from build123d import *

# Parameters (mm, degrees)
ESBO_O1_W                = 3
ESBO_O1_H                = 3
RESSALTO_EXTRUS_O1_DEPTH = 230


with BuildPart() as part:
    # Esboço1 → Ressalto-extrusão1 (new, symmetric)
    with BuildSketch(Plane.XY):
        with BuildLine():
            Line((15, 13.5), (15, 4.05))
            Line((15, 4.05), (13, 4.05))
            Line((13, 4.05), (13, 9))
            Line((13, 9), (10.414213562, 9))
            Line((10.414213562, 9), (7.9, 6.485786438))
            Line((7.9, 6.485786438), (7.9, -7.36e-07))
            Line((7.9, -7.36e-07), (7.9, -6.485786438))
            Line((7.9, -6.485786438), (10.414213562, -9))
            Line((10.414213562, -9), (13, -9))
            Line((13, -9), (13, -4.05))
            Line((13, -4.05), (15, -4.05))
            Line((15, -4.05), (15, -13.5))
            ThreePointArc((15, -13.5), (14.560660172, -14.560660172), (13.5, -15))
            Line((13.5, -15), (4.05, -15))
            Line((4.05, -15), (4.05, -13))
            Line((4.05, -13), (9, -13))
            Line((9, -13), (9, -10.414213562))
            Line((9, -10.414213562), (6.485786438, -7.9))
            Line((6.485786438, -7.9), (-7.36e-07, -7.9))
            Line((-7.36e-07, -7.9), (-6.485786438, -7.9))
            Line((-6.485786438, -7.9), (-9, -10.414213562))
            Line((-9, -10.414213562), (-9, -13))
            Line((-9, -13), (-4.05, -13))
            Line((-4.05, -13), (-4.05, -15))
            Line((-4.05, -15), (-13.5, -15))
            ThreePointArc((-13.5, -15), (-14.560660172, -14.560660172), (-15, -13.5))
            Line((-15, -13.5), (-15, -4.05))
            Line((-15, -4.05), (-13, -4.05))
            Line((-13, -4.05), (-13, -9))
            Line((-13, -9), (-10.414213562, -9))
            Line((-10.414213562, -9), (-7.9, -6.485786438))
            Line((-7.9, -6.485786438), (-7.9, 7.36e-07))
            Line((-7.9, 7.36e-07), (-7.9, 6.485786438))
            Line((-7.9, 6.485786438), (-10.414213562, 9))
            Line((-10.414213562, 9), (-13, 9))
            Line((-13, 9), (-13, 4.05))
            Line((-13, 4.05), (-15, 4.05))
            Line((-15, 4.05), (-15, 13.5))
            ThreePointArc((-15, 13.5), (-14.560660172, 14.560660172), (-13.5, 15))
            Line((-13.5, 15), (-4.05, 15))
            Line((-4.05, 15), (-4.05, 13))
            Line((-4.05, 13), (-9, 13))
            Line((-9, 13), (-9, 10.414213562))
            Line((-9, 10.414213562), (-6.485786438, 7.9))
            Line((-6.485786438, 7.9), (7.36e-07, 7.9))
            Line((7.36e-07, 7.9), (6.485786438, 7.9))
            Line((6.485786438, 7.9), (9, 10.414213562))
            Line((9, 10.414213562), (9, 13))
            Line((9, 13), (4.05, 13))
            Line((4.05, 13), (4.05, 15))
            Line((4.05, 15), (13.5, 15))
            ThreePointArc((13.5, 15), (14.560660172, 14.560660172), (15, 13.5))
        make_face()
        with Locations((-11.5, 11.5)):
            Rectangle(ESBO_O1_W, ESBO_O1_H, mode=Mode.SUBTRACT)
        with BuildLine():
            Line((-6.9, 1.000000736), (-6.9, 7.36e-07))
            Line((-6.9, 7.36e-07), (-6.9, -1.000000736))
            Line((-6.9, -1.000000736), (-5.966782929, -1.000000736))
            ThreePointArc((-5.966782929, -1.000000736), (-5.665339038, -2.122836212), (-5.154690025, -3.167281286))
            Line((-5.154690025, -3.167281286), (-6.9, -4.91259126))
            Line((-6.9, -4.91259126), (-6.9, -5.827922061))
            Line((-6.9, -5.827922061), (-5.827922061, -6.9))
            Line((-5.827922061, -6.9), (-4.91259126, -6.9))
            Line((-4.91259126, -6.9), (-3.167281286, -5.154690025))
            ThreePointArc((-3.167281286, -5.154690025), (-2.122836212, -5.665339038), (-1.000000736, -5.966782929))
            Line((-1.000000736, -5.966782929), (-1.000000736, -6.9))
            Line((-1.000000736, -6.9), (-7.36e-07, -6.9))
            Line((-7.36e-07, -6.9), (1.000000736, -6.9))
            Line((1.000000736, -6.9), (1.000000736, -5.966782929))
            ThreePointArc((1.000000736, -5.966782929), (2.122836212, -5.665339038), (3.167281286, -5.154690025))
            Line((3.167281286, -5.154690025), (4.91259126, -6.9))
            Line((4.91259126, -6.9), (5.827922061, -6.9))
            Line((5.827922061, -6.9), (6.9, -5.827922061))
            Line((6.9, -5.827922061), (6.9, -4.91259126))
            Line((6.9, -4.91259126), (5.154690025, -3.167281286))
            ThreePointArc((5.154690025, -3.167281286), (5.665339038, -2.122836212), (5.966782929, -1.000000736))
            Line((5.966782929, -1.000000736), (6.9, -1.000000736))
            Line((6.9, -1.000000736), (6.9, -7.36e-07))
            Line((6.9, -7.36e-07), (6.9, 1.000000736))
            Line((6.9, 1.000000736), (5.966782929, 1.000000736))
            ThreePointArc((5.966782929, 1.000000736), (5.665339038, 2.122836212), (5.154690025, 3.167281286))
            Line((5.154690025, 3.167281286), (6.9, 4.91259126))
            Line((6.9, 4.91259126), (6.9, 5.827922061))
            Line((6.9, 5.827922061), (5.827922061, 6.9))
            Line((5.827922061, 6.9), (4.91259126, 6.9))
            Line((4.91259126, 6.9), (3.167281286, 5.154690025))
            ThreePointArc((3.167281286, 5.154690025), (2.122836212, 5.665339038), (1.000000736, 5.966782929))
            Line((1.000000736, 5.966782929), (1.000000736, 6.9))
            Line((1.000000736, 6.9), (7.36e-07, 6.9))
            Line((7.36e-07, 6.9), (-1.000000736, 6.9))
            Line((-1.000000736, 6.9), (-1.000000736, 5.966782929))
            ThreePointArc((-1.000000736, 5.966782929), (-2.122836212, 5.665339038), (-3.167281286, 5.154690025))
            Line((-3.167281286, 5.154690025), (-4.91259126, 6.9))
            Line((-4.91259126, 6.9), (-5.827922061, 6.9))
            Line((-5.827922061, 6.9), (-6.9, 5.827922061))
            Line((-6.9, 5.827922061), (-6.9, 4.91259126))
            Line((-6.9, 4.91259126), (-5.154690025, 3.167281286))
            ThreePointArc((-5.154690025, 3.167281286), (-5.665339038, 2.122836212), (-5.966782929, 1.000000736))
            Line((-5.966782929, 1.000000736), (-6.9, 1.000000736))
        make_face(mode=Mode.SUBTRACT)
        with Locations((11.5, 11.5)):
            Rectangle(ESBO_O1_W, ESBO_O1_H, mode=Mode.SUBTRACT)
        with Locations((11.5, -11.5)):
            Rectangle(ESBO_O1_W, ESBO_O1_H, mode=Mode.SUBTRACT)
        with Locations((-11.5, -11.5)):
            Rectangle(ESBO_O1_W, ESBO_O1_H, mode=Mode.SUBTRACT)
    extrude(amount=RESSALTO_EXTRUS_O1_DEPTH, both=True)


solid = part.part
Geometry check sheet. Reference: the model listing, model coordinates, mm. A direction names the side the tool comes from. Round coordinates to 2 decimals unless told otherwise and drop trailing zeros. Use one line per item in the form item = value.
1. Scan lines: line 1 along Y through (x, z) = (12.75, -48); line 2 along X through (y, z) = (-7.5, -74). Record each from-to range of solid material in increasing order. Write a range as from..to.
Working result:
line_1 = -15..-13, -10..-9, 9..10, 13..15
line_2 = -15..-13, -8.91..8.91, 13..15
2. Cross-section at A-A, the plane z = 196. Count the separate pieces of the cut face and the enclosed holes in it, plus the area to 3 significant figures.
Working result:
separate_pieces = 1
enclosed_holes = 5
area = 301 mm^2
3. Go/stop test with flat-tipped pins: pin 1 (1.6 mm diameter, centred on x = 14, z = 30.5, fed in from +Y); pin 2 (1.5 mm diameter, centred on y = 1.5, z = 178, fed in from -X); pin 3 (2 mm diameter, centred on x = -1.5, z = -51.5, fed in from +Y); pin 4 (4 mm diameter, centred on y = -0.5, z = -96.5, fed in from +X). Record where each tip stops, or that it passes through.
Working result:
pin_1 = 15
pin_2 = -7.9
pin_3 = 7.9
pin_4 = 7.9
4. Mould release check, pull along Z, two halves, no side actions. Record for faces 3 (the face through (-6, -3, -230)), 4 (the face through (0, -7.9, 3)), 5 (the face through (-6, -3, 230)): pulls with the +Z half, pulls with the -Z half, needs draft (parallel to the pull), parting line crosses it, or undercut.
Working result:
face_3 = pulls with the -Z half
face_4 = needs draft
face_5 = pulls with the +Z half
5. Set-up check for faces 1 (the face through (-9, -15, 3)), 2 (the face through (-7.9, 0, 3)): record each of +Z, -Z, +X, -X, +Y, -Y from which the full face is reachable in a straight line by a thin tool's end or side.
Working result:
face_1 = +Z, -Z, +X, -X, -Y
face_2 = +Z, -Z
